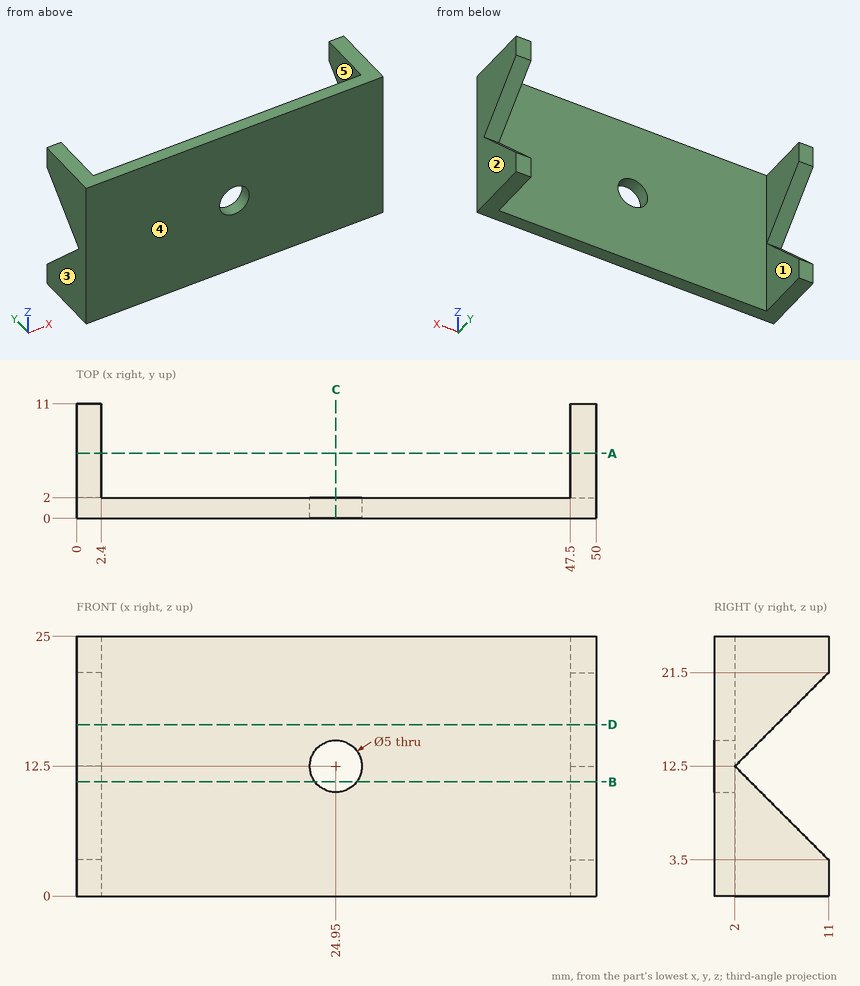
Job drawing, mm, ordinate dimensions from the low corner. One solid piece. A direction names the side the tool comes from. Coordinates: 2 decimals unless noted, no trailing zeros. Write each loop counter-clockwise with the first axis right and the second up, starting at its lowest first coordinate (ties: lowest second). Pieces come first, ordered by that corner, then holes.
Item 1: Slice it at A-A (y = 6.25). Write the cut outline in (x, z).
Item 2: Probe line 1 (X direction, y = 1.5, z = 12.5); line 2 (Z direction, x = 24.95, y = 0.9); line 3 (X direction, y = 4.75, z = 7). List the from-to ranges inside material, lowest first.
Item 3: Pin check, flat tips, straight feed: pin 1 (1 mm diameter, centred on y = 2.5, z = 12.5, fed in from +X); pin 2 (7.5 mm diameter, centred on x = 26, z = 15, fed in from +Y); pin 3 (5 mm diameter, centred on y = 7, z = 11.5, fed in from +X). Stop position of each tip, or through.
Item 4: Slice it at C-C (x = 24.95). Write the cut outline in (y, z), and give its area (3 significant figures).
Item 5: Slice it at D-D (z = 16.5). Write the cut outline in (x, y), and give its area (3 significant figures).
Item 6: Mould opens along X. For the marked faces 1, 2 and 3 say: released by +X, released by -X, zero draft, split by the parting line, or undercut.
Item 7: Slice it at B-B (z = 11). Write the cut outline in (x, y).
Item 8: Which spindle directions (+Z, -Z, +X, -X, +Y, -Y) get a long thin tool onto all of the face, cutting with end or side? Do the marked faces 4 and 5. Say none if no direction does.
Results found:
1. outline: (0, 0) - (2.4, 0) - (2.4, 8.25) - (0, 8.25) - close; (0, 16.75) - (2.4, 16.75) - (2.4, 25) - (0, 25) - close; (47.5, 0) - (50, 0) - (50, 8.25) - (47.5, 8.25) - close; (47.5, 16.75) - (50, 16.75) - (50, 25) - (47.5, 25) - close
2. line 1: x = 0 to 22.45, 27.45 to 50
2. line 2: z = 0 to 10, 15 to 25
2. line 3: x = 0 to 2.4, 47.5 to 50
3. pin 1: stops at x = 50
3. pin 2: stops at y = 2
3. pin 3: passes through
4. outline: (0, 0) - (2, 0) - (2, 10) - (0, 10) - close; (0, 15) - (2, 15) - (2, 25) - (0, 25) - close
4. area: 40.0 mm2
5. outline: (0, 0) - (50, 0) - (50, 6) - (47.5, 6) - (47.5, 2) - (2.4, 2) - (2.4, 6) - (0, 6) - close
5. area: 120 mm2
6. face 1: undercut
6. face 2: released by +X
6. face 3: released by -X
7. outline: (0, 0) - (22.95, 0) - (22.95, 2) - (2.4, 2) - (2.4, 3.5) - (0, 3.5) - close; (26.95, 0) - (50, 0) - (50, 3.5) - (47.5, 3.5) - (47.5, 2) - (26.95, 2) - close
8. face 4: +Z, -Z, +X, -X, -Y
8. face 5: +Z, -Z, +Y
